```python
from build123d import *

# Parameters (mm, degrees)
SKETCH1_W           = 130
SKETCH1_H           = 55
SKETCH1_R           = 1.6
SKETCH1_R_2         = 1.25
BOSS_EXTRUDE1_DEPTH = 3.5
FILLET1_R           = 10


with BuildPart() as part:
    # Sketch1 → Boss-Extrude1 (new body)
    with BuildSketch(Plane(origin=(0, 0, 0), x_dir=(1, 0, 0), z_dir=(0, 1, 0))):
        with Locations((65, -27.5)):
            Rectangle(SKETCH1_W, SKETCH1_H)
        with Locations((9, -12.5)):
            Circle(SKETCH1_R, mode=Mode.SUBTRACT)
        with Locations((9, -42.5)):
            Circle(SKETCH1_R, mode=Mode.SUBTRACT)
        with Locations((33, -12.5)):
            Circle(SKETCH1_R, mode=Mode.SUBTRACT)
        with Locations((33, -42.5)):
            Circle(SKETCH1_R, mode=Mode.SUBTRACT)
        with Locations((121, -42.5)):
            Circle(SKETCH1_R, mode=Mode.SUBTRACT)
        with Locations((97, -42.5)):
            Circle(SKETCH1_R, mode=Mode.SUBTRACT)
        with Locations((97, -12.5)):
            Circle(SKETCH1_R, mode=Mode.SUBTRACT)
        with Locations((121, -12.5)):
            Circle(SKETCH1_R, mode=Mode.SUBTRACT)
        with Locations((83.7, -8.8)):
            Circle(SKETCH1_R_2, mode=Mode.SUBTRACT)
        with Locations((83.7, -46.2)):
            Circle(SKETCH1_R_2, mode=Mode.SUBTRACT)
        with Locations((46.3, -46.2)):
            Circle(SKETCH1_R_2, mode=Mode.SUBTRACT)
        with Locations((46.3, -8.8)):
            Circle(SKETCH1_R_2, mode=Mode.SUBTRACT)
    extrude(amount=BOSS_EXTRUDE1_DEPTH)

    # Fillet1
    fillet1_edges = [part.edges().sort_by_distance(p)[0] for p in [
        (0, 1.75, 0),
        (130, 1.75, 0),
        (130, 1.75, 55),
        (0, 1.75, 55),
    ]]
    fillet(fillet1_edges, radius=FILLET1_R)


solid = part.part
```
Source: CAD feature listing. Evaluate the final solid. Frame: model axes, mm. Give positions to 0.01 mm unless a question says otherwise; leave off trailing zeros. Loops run counter-clockwise (first coordinate to the right, second up) from the corner with the lowest first, then second, coordinate; pieces in that order, holes last. Notation, with made-up numbers: (61.5, 3) - (84.5, 3) arc R33 cw to (84.5, 32) - close; hole circle Ø1 at (60, 5). An arc over 180 degrees is marked (long way). Use CSV: the item, a comma, the result in double quotes. Start each with the question number.
1. Ray query, L1, parallel to X at y = 0.7, z = 42.5; L2, parallel to Z at x = 97, y = 1; L3, parallel to Z at x = 83.7, y = 0.9. Return the intervals inside material, ascending.
2. Section A-A (z = 12.5). Output: boundary loops of the cut face in (x, y).
3. Pin query (flat end, axial travel): pin 1 (3 mm diameter, centred on x = 97, z = 12.5, fed in from +Y). Return the tip coordinate at first contact, or that it passes through.
4. Draft query along X for faces 1 (the cylindrical face through (95.4, 1.73, 42.43)), 2 (the flat face through (64, 2, 55)), 3 (the cylindrical face through (2.85, 1.77, 3.01)). Return one class per face: +X half, -X half, draft (parallel to the pull), parting line (faces both ways), or undercut.
5. Section C-C (y = 2.3). Count the separate pieces of the cut face and the enclosed holes in it, then the cut area to 3 significant figures.
6. Section B-B (x = 33). Output: boundary loops of the cut face in (y, z).
7. Section D-D (z = 46.2). Output: boundary loops of the cut face in (x, y), then the cut area to 3 significant figures.
Response:
1,L1,"0 to 7.4, 10.6 to 31.4, 34.6 to 95.4, 98.6 to 119.4, 122.6 to 130"
1,L2,"0 to 10.9, 14.1 to 40.9, 44.1 to 55"
1,L3,"0 to 7.55, 10.05 to 44.95, 47.45 to 55"
2,outline,"(0, 0) - (7.4, 0) - (7.4, 3.5) - (0, 3.5) - close; (10.6, 0) - (31.4, 0) - (31.4, 3.5) - (10.6, 3.5) - close; (34.6, 0) - (95.4, 0) - (95.4, 3.5) - (34.6, 3.5) - close; (98.6, 0) - (119.4, 0) - (119.4, 3.5) - (98.6, 3.5) - close; (122.6, 0) - (130, 0) - (130, 3.5) - (122.6, 3.5) - close"
3,pin 1,"through"
4,face 1,"undercut"
4,face 2,"draft"
4,face 3,"-X half"
5,separate pieces,"1"
5,enclosed holes,"12"
5,area,"6,980 mm²"
6,outline,"(0, 0) - (3.5, 0) - (3.5, 10.9) - (0, 10.9) - close; (0, 14.1) - (3.5, 14.1) - (3.5, 40.9) - (0, 40.9) - close; (0, 44.1) - (3.5, 44.1) - (3.5, 55) - (0, 55) - close"
7,outline,"(0.07, 0) - (45.05, 0) - (45.05, 3.5) - (0.07, 3.5) - close; (47.55, 0) - (82.45, 0) - (82.45, 3.5) - (47.55, 3.5) - close; (84.95, 0) - (129.93, 0) - (129.93, 3.5) - (84.95, 3.5) - close"
7,area,"437 mm²"
